Verification items for this drawing (mm, ordinates from the low corner). A direction names the side the tool comes from. Round coordinates to 2 decimals unless told otherwise and drop trailing zeros. Order: outer loops, then holes, each group sorted by start corner. A loop starts at its lowest first (then second) coordinate and runs counter-clockwise, first axis right, second up. Notation, with made-up numbers: (77.5, 34) -> (129.5, 34) arc R20 ccw to (129.5, 41) -> close; hole circle Ø11 at (-16.5, -11). An arc over 180 degrees is marked (long way). Answer in a Markdown table with one row per item. Add a question column.
1. Material ranges on L1, parallel to Y at x = 7, z = 6.5; L2, parallel to Y at x = 2.25, z = 3.25; L3, parallel to Z at x = 5.75, y = 16.75, recorded low to high. Write a range as from..to.
2. Draft check along X on the marked faces 3, 4 and 5. Enter one of: +X half, -X half, draft (parallel to the pull), parting line (faces both ways), or undercut.
3. Access from +Z, -Z, +X, -X, +Y, -Y to the whole of each face (thin tool, end or side, straight path). Record for the marked faces 1 and 2.
4. Sectioned sample at D-D, the plane x = 11.75. Record the boundary of the cut face in (y, z), then the cut area to 3 significant figures.
5. Sectioned sample at B-B, the plane x = 7.6. Record the boundary of the cut face in (y, z) (1 decimal), then the cut area to 3 significant figures.
6. Sectioned sample at A-A, the plane z = 7.6. Record the boundary of the cut face in (x, y) (1 decimal), then the cut area to 3 significant figures.
7. Depth check by flat-ended pin: P1, Ø8, axis at y = 10, z = 9.5, coming from the -X side (3 decimals); P2, Ø4, axis at x = 7.5, z = 10, coming from the -Y side; P3, Ø3, axis at x = 11.5, y = 20.5, coming from the +Z side (1 decimal); P4, Ø4, axis at x = 7, y = 14.5, coming from the +Z side (3 decimals). Enter the tip coordinate at first touch or a pass-through.
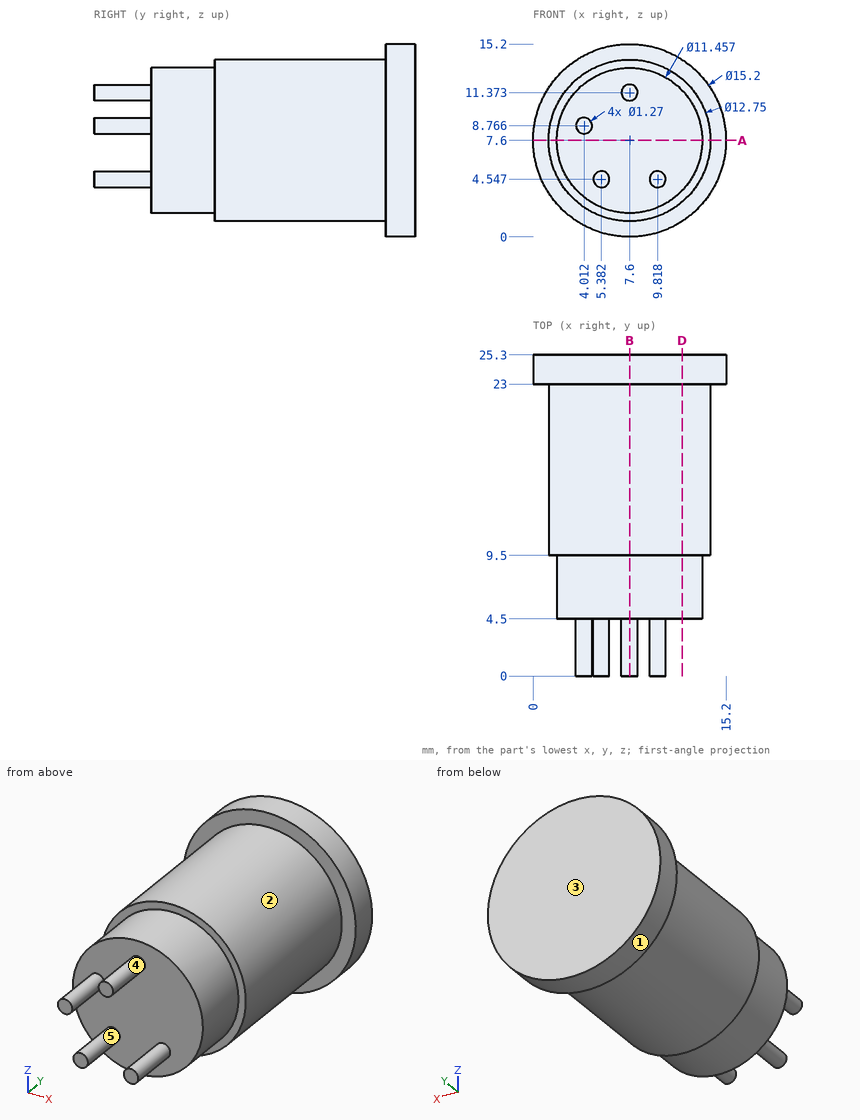
Answer key:
| question | item | result |
|---|---|---|
| 1 | L1 | y = 4.5..25.3 |
| 1 | L2 | y = 23..25.3 |
| 1 | L3 | z = 1.5..13.7 |
| 2 | face 3 | draft |
| 2 | face 4 | parting line |
| 2 | face 5 | undercut |
| 3 | face 1 | +Y, -Y |
| 3 | face 2 | -Y |
| 4 | outline | (4.5, 3.65) -> (9.5, 3.65) -> (9.5, 2.76) -> (23, 2.76) -> (23, 1.23) -> (25.3, 1.23) -> (25.3, 13.97) -> (23, 13.97) -> (23, 12.44) -> (9.5, 12.44) -> (9.5, 11.55) -> (4.5, 11.55) -> close |
| 4 | area | 199 mm² |
| 5 | outline | (0, 10.7) -> (4.5, 10.7) -> (4.5, 1.9) -> (9.5, 1.9) -> (9.5, 1.2) -> (23, 1.2) -> (23, 0) -> (25.3, 0) -> (25.3, 15.2) -> (23, 15.2) -> (23, 14) -> (9.5, 14) -> (9.5, 13.3) -> (4.5, 13.3) -> (4.5, 12) -> (0, 12) -> close |
| 5 | area | 270 mm² |
| 6 | outline | (0, 23) -> (1.2, 23) -> (1.2, 9.5) -> (1.9, 9.5) -> (1.9, 4.5) -> (13.3, 4.5) -> (13.3, 9.5) -> (14, 9.5) -> (14, 23) -> (15.2, 23) -> (15.2, 25.3) -> (0, 25.3) -> close |
| 6 | area | 264 mm² |
| 7 | P1 | stops at x = 1.225 |
| 7 | P2 | stops at y = 0 |
| 7 | P3 | stops at z = 13.5 |
| 7 | P4 | stops at z = 13.975 |
